Geometry check sheet. Reference: the model listing, model coordinates, mm. A direction names the side the tool comes from. Coordinates: 2 decimals unless noted, no trailing zeros. Loops run counter-clockwise (first coordinate to the right, second up) from the corner with the lowest first, then second, coordinate; pieces in that order, holes last. Notation, with made-up numbers: (4, 14) - (54, 14) arc R9 cw to (54, 29) - close; hole circle Ø7 at (33, 47). An arc over 180 degrees is marked (long way). One line per item, written item: value.
from build123d import *

# Parameters (mm, degrees)
SKETCH1_W           = 63.5
SKETCH1_H           = 50.8
BOSS_EXTRUDE1_DEPTH = 6.35
BOSS_EXTRUDE2_DEPTH = 28.575
SKETCH4_R           = 2.25
CUT_EXTRUDE2_DEPTH  = 7.35
FILLET1_R           = 2.54
SKETCH5_R           = 2.413
CUT_EXTRUDE3_DEPTH  = 39.823652545
BOSS_EXTRUDE3_DEPTH = 6.35
SKETCH7_R           = 5.588
CUT_EXTRUDE4_DEPTH  = 32.823641145


with BuildPart() as part:
    # Sketch1 → Boss-Extrude1 (new body)
    with BuildSketch(Plane(origin=(0, 0, 0), x_dir=(1, 0, 0), z_dir=(0, 1, 0))):
        Rectangle(SKETCH1_W, SKETCH1_H)
    extrude(amount=BOSS_EXTRUDE1_DEPTH)

    # Sketch2 → Boss-Extrude2 (add)
    with BuildSketch(Plane(origin=(0, 6.35, 0), x_dir=(1, 0, 0), z_dir=(0, 1, 0))):
        Polygon((2.907968577, -15.052543666), (-15.052543666, 2.907968577), (-10.102788136, 7.857724106), (7.857724106, -10.102788136), align=None)
    extrude(amount=BOSS_EXTRUDE2_DEPTH)

    # Sketch4 → Cut-Extrude2 (cut, through all)
    with BuildSketch(Plane(origin=(0, 6.35, 0), x_dir=(1, 0, 0), z_dir=(0, 1, 0))):
        with Locations((10, -19.85)):
            Circle(SKETCH4_R)
        with Locations((10, 19.85)):
            Circle(SKETCH4_R)
        with Locations((-10, 19.85)):
            Circle(SKETCH4_R)
        with Locations((-10, -19.85)):
            Circle(SKETCH4_R)
    extrude(amount=-CUT_EXTRUDE2_DEPTH, mode=Mode.SUBTRACT)

    # Fillet1
    fillet1_edges = [part.edges().sort_by_distance(p)[0] for p in [
        (5.382846341, 6.35, 12.577665901),
        (-12.577665901, 6.35, -5.382846341),
        (5.382846341, 34.925, 12.577665901),
        (-12.577665901, 34.925, -5.382846341),
    ]]
    fillet(fillet1_edges, radius=FILLET1_R)

    # Sketch5 → Cut-Extrude3 (cut, through all)
    with BuildSketch(Plane(origin=(-1.122532015, 0, 1.122532015), x_dir=(-0.707106781, 0, -0.707106781), z_dir=(0.707106781, 0, -0.707106781))):
        with Locations((0, 22.225)):
            Circle(SKETCH5_R)
    extrude(amount=-CUT_EXTRUDE3_DEPTH, mode=Mode.SUBTRACT)

    # Sketch6 → Boss-Extrude3 (add, symmetric)
    with BuildSketch(Plane(origin=(0, 0, 0), x_dir=(-0.707106781, 0, 0.707106781), z_dir=(-0.707106781, 0, -0.707106781))):
        Polygon((8.5875114, 34.925), (14.9375114, 6.35), (8.5875114, 6.35), align=None)
    extrude(amount=BOSS_EXTRUDE3_DEPTH, both=True)

    # Sketch7 → Cut-Extrude4 (cut, through all)
    with BuildSketch(Plane(origin=(-6.072287544, 0, 6.072287544), x_dir=(0.707106781, 0, 0.707106781), z_dir=(-0.707106781, 0, 0.707106781))):
        with Locations((0, 22.225)):
            Circle(SKETCH7_R)
    extrude(amount=CUT_EXTRUDE4_DEPTH, mode=Mode.SUBTRACT)


solid = part.part
(1) Access from +Z, -Z, +X, -X, +Y, -Y to the whole of each face (thin tool, end or side, straight path). Record for faces 1 (the face through (-1.273, 17.262, 0.972)), 2 (the face through (-12.61, 20.47, -5.35)), 3 (the face through (-12.963, 20.437, -0.818)).
Reply:
face 1: -Z, +X, +Y
face 2: -Z, -X, +Y
face 3: -X, +Y
(2) Cross-section at A-A on z = -19.85. Record the cut outline in (x, y), and give its area (3 significant figures).
Reply:
outline: (-31.75, 0) - (-12.25, 0) - (-12.25, 6.35) - (-31.75, 6.35) - close; (-7.75, 0) - (7.75, 0) - (7.75, 6.35) - (-7.75, 6.35) - close; (12.25, 0) - (31.75, 0) - (31.75, 6.35) - (12.25, 6.35) - close
area: 346 mm2
(3) Cross-section at B-B on y = 3.5. Record the cut outline in (x, z), and give its area (3 significant figures).
Reply:
outline: (-31.75, -25.4) - (31.75, -25.4) - (31.75, 25.4) - (-31.75, 25.4) - close; hole circle Ø4.5 at (-10, -19.85); hole circle Ø4.5 at (-10, 19.85); hole circle Ø4.5 at (10, -19.85); hole circle Ø4.5 at (10, 19.85)
area: 3,160 mm2
(4) Material ranges on probe 1 along Z at (x, y) = (10, 2.5); probe 2 along X at (y, z) = (2.75, 19.85); probe 3 along X at (y, z) = (3, -21.5), recorded low to high. Write a range as from..to.
Reply:
probe 1: -25.4..-22.1, -17.6..17.6, 22.1..25.4
probe 2: -31.75..-12.25, -7.75..7.75, 12.25..31.75
probe 3: -31.75..-11.53, -8.47..8.47, 11.53..31.75
(5) Release check for a two-part mould opening along Z. For faces 4 (the face through (-11.84, 14.49, 2.86)), 5 (the face through (0, 0, 0)), 6 (the face through (0, 3, 25.4)) record: pulls with the +Z half, pulls with the -Z half, needs draft (parallel to the pull), parting line crosses it, or undercut.
Reply:
face 4: undercut
face 5: needs draft
face 6: pulls with the +Z half
(6) Cross-section at C-C on x = 25. Record the cut outline in (y, z).
Reply:
outline: (0, -25.4) - (6.35, -25.4) - (6.35, 25.4) - (0, 25.4) - close
(7) Cross-section at D-D on z = -14. Record the cut outline in (x, y), and give its area (3 significant figures).
Reply:
outline: (-31.75, 0) - (31.75, 0) - (31.75, 6.35) - (-31.75, 6.35) - close
area: 403 mm2
(8) Go/stop test with flat-tipped pins: pin 1 Ø8 at (x, z) = (25, -7.5) entering from +Y; pin 2 Ø8 at (x, y) = (-10.5, 11.5) entering from +Z; pin 3 Ø10 at (x, y) = (8, 29.5) entering from -Z. Record where each tip stops, or that it passes through.
Reply:
pin 1: y = 6.35
pin 2: z = 13.2
pin 3: z = 5.25
